For this review, take the finished solid that the model builds, in its own axes (mm). A direction names the side the tool comes from. Round coordinates to 2 decimals unless told otherwise and drop trailing zeros. Write each loop counter-clockwise with the first axis right and the second up, starting at its lowest first coordinate (ties: lowest second). Pieces come first, ordered by that corner, then holes. Notation, with made-up numbers: M -13,21 L 20,21 A29 cw 20,55 Z; hole C 52.25,21 d3. An arc over 180 degrees is marked long. Use one line per item in the form item = value. Start each with the question number.
Item 1: For P1, Ø4, axis at x = 15.5, z = 44, coming from the -Y side; P2, Ø3, axis at x = 5.08, z = 5.08, coming from the -Y side; P3, Ø6, axis at x = 7, z = 6.5, coming from the -Y side; P4, Ø6, axis at x = 52.07, z = 52.07, coming from the +Y side, all flat-tipped, find the tip position at first contact; note any pin that passes through.
Item 2: Add section B-B (x = 21). State the section outline as (y, z) points, and give its area (3 significant figures).
Item 3: Add section A-A (y = -110). State the section outline as (x, z) points.
Item 4: For line 1 (X direction, y = -108, z = 52), list the stretches that pass through material, from the lowest coordinate up. Write a range as [from, to].
Item 5: For faces 1 (the flat face through (57.15, -57, 28)), 2 (the flat face through (52, -89.916, 5)), list the 3-axis set-ups (+Z, -Z, +X, -X, +Y, -Y) from which the entire face can be reached by the end or side of a thin tool; tool diameter is ignored.
Item 6: Draft analysis for pull direction X (two halves, no side actions). For faces 3 (the cylindrical face through (6.311, -102.794, 2.714)), 4 (the flat face through (0, -57, 28)), 5 (the flat face through (28, 0, 29)), state which applies: released by +X, released by -X, zero draft, split by the parting line, or undercut.
Item 7: Add section C-C (z = 13.5). State the section outline as (x, y) points, and give its area (3 significant figures).
from build123d import *

# Parameters (mm, degrees)
F0_W     = 57.15
F0_H     = 57.15
F1_DEPTH = 115.316
F2_R     = 5.08
F3_R     = 19.05
F4_DEPTH = 1.524
F5_R     = 3.175
F6_DEPTH = 19.05
F7_R     = 2.667
F8_DEPTH = 25.4


with BuildPart() as f1:
    # F0 (on Front) → F1 (new body)
    with BuildSketch(Plane.XZ):
        with Locations((28.575, 28.575)):
            Rectangle(F0_W, F0_H)
    extrude(amount=F1_DEPTH)

    # F2
    f2_edges = [f1.edges().sort_by_distance(p)[0] for p in [
        (57.15, -57.658, 57.15),
        (57.15, -57.658, 0),
        (0, -57.658, 0),
        (0, -57.658, 57.15),
    ]]
    fillet(f2_edges, radius=F2_R)

    # F3 (on face) → F4 (join)
    with BuildSketch(Plane.XZ.offset(115.316)):
        with Locations((28.575, 28.575)):
            Circle(F3_R)
    extrude(amount=F4_DEPTH)

    # F5 (on face) → F6 (join)
    with BuildSketch(Plane.XZ.offset(116.84)):
        with Locations((28.575, 28.575)):
            Circle(F5_R)
    extrude(amount=F6_DEPTH)

    # F7 (on face) → F8 (cut)
    with BuildSketch(Plane.XZ.offset(115.316)):
        with Locations((52.07, 52.07)):
            Circle(F7_R)
        with Locations((5.08, 52.07)):
            Circle(F7_R)
        with Locations((52.07, 5.08)):
            Circle(F7_R)
        with Locations((5.08, 5.08)):
            Circle(F7_R)
    extrude(amount=-F8_DEPTH, mode=Mode.SUBTRACT)


solid = f1.part
Calculated:
q1.P1 = -116.84
q1.P2 = -89.92
q1.P3 = -115.32
q1.P4 = 0
q2.outline = M -116.84,11.1 L -115.32,11.1 L -115.32,0 L 0,0 L 0,57.15 L -115.32,57.15 L -115.32,46.05 L -116.84,46.05 Z
q2.area = 6,640 mm^2
q3.outline = M 0,5.08 A5.08 ccw 5.08,0 L 52.07,0 A5.08 ccw 57.15,5.08 L 57.15,52.07 A5.08 ccw 52.07,57.15 L 5.08,57.15 A5.08 ccw 0,52.07 Z; hole C 5.08,5.08 d5.33; hole C 5.08,52.07 d5.33; hole C 52.07,5.08 d5.33; hole C 52.07,52.07 d5.33
q4.line_1 = [0, 2.41], [7.75, 49.4], [54.74, 57.15]
q5.face_1 = +Z, -Z, +X, +Y, -Y
q5.face_2 = -Y
q6.face_3 = undercut
q6.face_4 = released by -X
q6.face_5 = zero draft
q7.outline = M 0,-115.32 L 16.93,-115.32 L 16.93,-116.84 L 40.22,-116.84 L 40.22,-115.32 L 57.15,-115.32 L 57.15,0 L 0,0 Z
q7.area = 6,630 mm^2
